Autodesk Inventor part; units mm, degrees
ref_plane "YZ Plane" through (0, 0, 0) normal (1, 0, 0) x (0, 1, 0)
ref_plane "XZ Plane" through (0, 0, 0) normal (0, 1, 0) x (-1, 0, 0)
ref_plane "XY Plane" through (0, 0, 0) normal (0, 0, 1) x (1, 0, 0)
sketch "スケッチ1" plane through (0, 0, 0) normal (0, 1, 0) x (-1, 0, 0)
  line L0 (0, 0) -> (-47.5, 0)
  line L1 (-47.5, 0) -> (-47.5, -47.5)
  line L2 (-47.5, -47.5) -> (0, -47.5)
  line L3 (0, -47.5) -> (0, 0)
  dimension "d0" = 47.5
  dimension "d1" = 47.5
extrude "押し出し1" add sketch "スケッチ1" along normal blind 28.4
ref_plane "作業平面1" through (0, 28.4, 0) normal (0, 1, 0) x (1, 0, 0)
sketch "スケッチ3" plane through (0, 28.4, 0) normal (0, 1, 0) x (1, 0, 0)
  line L0 (3, 3) -> (44.5, 3)
  line L1 (44.5, 3) -> (44.5, 44.5)
  line L2 (44.5, 44.5) -> (3, 44.5)
  line L3 (3, 44.5) -> (3, 3)
  line L4 (47.5, 47.5) -> (0, 47.5)
  line L5 (0, 47.5) -> (0, 0)
  dimension "d15" = 41.5
  dimension "d16" = 41.5
  dimension "d17" = 3
  dimension "d18" = 3
extrude "押し出し3" cut sketch "スケッチ3" against normal blind 23.6
ref_plane "作業平面2" through (0, 4.8, 0) normal (0, 1, 0) x (1, 0, 0)
sketch "スケッチ4" plane through (0, 4.8, 0) normal (0, 1, 0) x (1, 0, 0)
  point P0 (0, 0)
  point P1 (23.75, 23.75)
hole "穴1" at (23.75, 4.8, -23.75) direction (0, -1, 0) diameter 22.5 end through all
sketch "スケッチ5" plane through (0, 4.8, 0) normal (0, 1, 0) x (1, 0, 0)
  line L0 (3, 44.5) -> (44.5, 44.5)
  line L1 (3, 3) -> (3, 44.5)
  line L2 (44.5, 44.5) -> (44.5, 3)
  line L3 (44.5, 3) -> (3, 3)
  point P0 (0, 0)
  point P1 (8.25, 39.25)
  point P2 (39.25, 39.25)
  point P3 (39.25, 8.25)
  point P4 (8.25, 8.25)
  dimension "d29" = 5.25
  dimension "d30" = 5.25
  dimension "d31" = 5.25
  dimension "d32" = 5.25
  dimension "d33" = 5.25
  dimension "d34" = 5.25
  dimension "d35" = 5.25
  dimension "d36" = 5.25
hole "穴2" at (8.25, 4.8, -39.25) at (39.25, 4.8, -39.25) at (39.25, 4.8, -8.25) at (8.25, 4.8, -8.25) direction (0, -1, 0) diameter 3.5 end through all
ref_plane "作業平面3" through (0, 0, 0) normal (0, 0, 1) x (1, 0, 0)
sketch "スケッチ6" plane through (0, 0, 0) normal (0, 0, 1) x (1, 0, 0)
  line L0 (16, 28.2) -> (31.5, 28.2)
  line L1 (31.5, 28.2) -> (31.5, 19.9)
  line L2 (31.5, 19.9) -> (16, 19.9)
  line L3 (16, 19.9) -> (16, 28.2)
  line L4 (0, 0) -> (47.5, 0)
  line L5 (0, 28.4) -> (47.5, 28.4)
  point P0 (23.75, 19.9)
  point P1 (23.75, 0)
  point P2 (23.75, 0)
  dimension "d46" = 19.9
  dimension "d47" = 0
  dimension "d48" = 15.5
  dimension "d51" = 8.5
extrude "押し出し4" cut sketch "スケッチ6" against normal blind 23.6
properties part number "motor_case"
Design review of the part built by this model. Coordinates are the model's own, in mm. A direction names the side the tool comes from. Round coordinates to 2 decimals unless told otherwise and drop trailing zeros. Order: outer loops, then holes, each group sorted by start corner. A loop starts at its lowest first (then second) coordinate and runs counter-clockwise, first axis right, second up. Notation, with made-up numbers: (20.25, 15) - (73.25, 15) arc R6 ccw to (73.25, 26) - close; hole circle Ø1 at (22.25, 5). An arc over 180 degrees is marked (long way). One line per question, with ' | ' between items.
Item 1: Take a section at C-C, the plane z = -23.75. Write out the cut boundary in (x, y), then the cut area to 3 significant figures.
Checks:
outline: (0, 0) - (12.5, 0) - (12.5, 4.8) - (3, 4.8) - (3, 28.4) - (0, 28.4) - close; (35, 0) - (47.5, 0) - (47.5, 28.4) - (44.5, 28.4) - (44.5, 4.8) - (35, 4.8) - close | area: 262 mm²
Item 2: For P1, Ø5.5, axis at x = 8.25, z = -8.25, coming from the +Y side, flat-tipped, find the tip position at first contact; note if it passes through.
Checks:
P1: y = 4.8
Item 3: Wall thickness on line 1 (X direction, y = 2.65, z = -8.25); line 2 (Z direction, x = 39.25, y = 3.1); line 3 (Z direction, x = 40.5, y = 7.75): over which ranges is each line inside the solid? List them lowest first. Write a range as [from, to].
Checks:
line 1: [0, 6.5], [10, 37.5], [41, 47.5] | line 2: [-47.5, -41], [-37.5, -10], [-6.5, 0] | line 3: [-47.5, -44.5], [-3, 0]
Item 4: Draft analysis for pull direction Z (two halves, no side actions). For faces 4 (the face through (47.5, 14, -23)), 5 (the face through (23, 14, 0)), 6 (the face through (40.96, 2.37, -8.63)), state which applies: +Z half, -Z half, draft (parallel to the pull), parting line (faces both ways), or undercut.
Checks:
face 4: draft | face 5: +Z half | face 6: undercut
Item 5: Take a section at B-B, the plane x = 23.75. Write out the cut boundary in (y, z), then the cut area to 3 significant figures.
Checks:
outline: (0, -47.5) - (28.4, -47.5) - (28.4, -44.5) - (4.8, -44.5) - (4.8, -35) - (0, -35) - close; (0, -12.5) - (4.8, -12.5) - (4.8, -3) - (19.9, -3) - (19.9, 0) - (0, 0) - close; (28.2, -3) - (28.4, -3) - (28.4, 0) - (28.2, 0) - close | area: 237 mm²
Item 6: Take a section at A-A, the plane y = 2.25. Write out the cut boundary in (x, z), then the cut area to 3 significant figures.
Checks:
outline: (0, -47.5) - (47.5, -47.5) - (47.5, 0) - (0, 0) - close; hole circle Ø3.5 at (8.25, -39.25); hole circle Ø3.5 at (8.25, -8.25); hole circle Ø22.5 at (23.75, -23.75); hole circle Ø3.5 at (39.25, -39.25); hole circle Ø3.5 at (39.25, -8.25) | area: 1,820 mm²
Item 7: Machinability: for faces 1 (the face through (16, 24, -1)), 2 (the face through (8.92, 2.366, -6.633)), 3 (the face through (23, 17, -3)), which of the approach directions +Z, -Z, +X, -X, +Y, -Y give a long, thin tool a straight path to every point of the face, cutting with its end or side? Answer none if there is none.
Checks:
face 1: +Z | face 2: +Y, -Y | face 3: +Y
Item 8: Take a section at D-D, the plane y = 23.25. Write out the cut boundary in (x, z).
Checks:
outline: (0, -47.5) - (47.5, -47.5) - (47.5, 0) - (31.5, 0) - (31.5, -3) - (44.5, -3) - (44.5, -44.5) - (3, -44.5) - (3, -3) - (16, -3) - (16, 0) - (0, 0) - close
